Work out the finished part from the listing and answer in its coordinate system (mm). Give positions to 0.01 mm unless a question says otherwise; leave off trailing zeros. Loops run counter-clockwise (first coordinate to the right, second up) from the corner with the lowest first, then second, coordinate; pieces in that order, holes last. Notation, with made-up numbers: (20.25, -37) - (39.25, -37) arc R17 ccw to (39.25, -16) - close; hole circle Ø9 at (66.25, -3). An arc over 180 degrees is marked (long way). One line per question, with ' | ' between items. Start each with the question number.
1. For a pull along X with two mould halves and no side action, classify faces 1 (the face through (-17, -2, 0)), 2 (the face through (17, -2, 0)), 3 (the face through (-16.7, -12, 0)) as released by +X, released by -X, zero draft, split by the parting line, or undercut.
2. Section A-A (y = -14.25) is taken. Determine the outline of the cut face in (x, z), plus the area to 3 significant figures.
3. Section B-B (z = 0) is taken. Determine the outline of the cut face in (x, y), plus the area to 3 significant figures.
4. Section C-C (x = -7) is taken. Determine the outline of the cut face in (y, z).
5. Each of these flat-tipped pins is pushed along its axis until it touches: pin 1 (1 mm diameter, centred on x = -2, z = -6.5, fed in from +Y); pin 2 (1 mm diameter, centred on x = -13.5, y = -6, fed in from +Z); pin 3 (8 mm diameter, centred on x = -6.5, z = -2.5, fed in from +Y); pin 4 (3 mm diameter, centred on x = 5.5, z = 4.5, fed in from +Y). Where does it stop, or does it pass through?
6. Find the intervals of material crossed by line 1 (Y direction, x = 1.5, z = -3.75); line 2 (Z direction, x = -3, y = -0.5); line 3 (Y direction, x = -10, z = -6.5), in increasing order.
from build123d import *

# Parameters (mm, degrees)
SKETCH_1_R      = 8.35
EXTRUDE_1_DEPTH = 17
FILLET_1_R      = 1
SKETCH_2_W      = 3
SKETCH_2_H      = 16.35
EXTRUDE_2_DEPTH = 0.3


with BuildPart() as part:
    # Эскиз1 → Бобышка-Вытянуть1 (new, symmetric)
    with BuildSketch(Plane(origin=(0, 0, 0), x_dir=(0, 0, -1), z_dir=(1, 0, 0))):
        Circle(SKETCH_1_R)
    extrude(amount=EXTRUDE_1_DEPTH, both=True)

    # Скругление1
    fillet_1_edges = [part.edges().sort_by_distance(p)[0] for p in [
        (-17, 0, 8.35),
        (17, 0, 8.35),
    ]]
    fillet(fillet_1_edges, radius=FILLET_1_R)

    # Эскиз2 → Бобышка-Вытянуть2 (add)
    with BuildSketch(Plane(origin=(17, 0, 0), x_dir=(0, 0, -1), z_dir=(1, 0, 0))):
        with Locations((0, -8.175)):
            Rectangle(SKETCH_2_W, SKETCH_2_H)
    extrude_2 = extrude(amount=-EXTRUDE_2_DEPTH)

    # Зеркальное отражение1: Бобышка-Вытянуть2 across plane
    add(extrude_2.mirror(Plane(origin=(0, 0, 0), x_dir=(0, 0, 1), z_dir=(1, 0, 0))))


solid = part.part
Conclusion:
1) face 1: released by -X | face 2: released by +X | face 3: undercut
2) outline: (-17, -1.5) - (-16.7, -1.5) - (-16.7, 1.5) - (-17, 1.5) - close; (16.7, -1.5) - (17, -1.5) - (17, 1.5) - (16.7, 1.5) - close | area: 1.80 mm²
3) outline: (-17, -16.35) - (-16.7, -16.35) - (-16.7, -8.06) arc R1 ccw to (-16, -8.35) - (16, -8.35) arc R1 ccw to (16.7, -8.06) - (16.7, -16.35) - (17, -16.35) - (17, 7.35) arc R1 ccw to (16, 8.35) - (-16, 8.35) arc R1 ccw to (-17, 7.35) - close | area: 572 mm²
4) outline: circle Ø16.7 at (0, 0)
5) pin 1: y = 5.81 | pin 2: z = 6.28 | pin 3: y = 8.35 | pin 4: y = 7.79
6) line 1: -7.46 to 7.46 | line 2: -8.34 to 8.34 | line 3: -5.24 to 5.24
